Work out the finished part from the listing and answer in its coordinate system (mm). A direction names the side the tool comes from. Give positions to 0.01 mm unless a question says otherwise; leave off trailing zeros. Loops run counter-clockwise (first coordinate to the right, second up) from the corner with the lowest first, then second, coordinate; pieces in that order, holes last. Notation, with made-up numbers: M -32,53 L -22,53 A22 ccw -22,92 Z; hole C -23,23.5 d2. An arc over 180 degrees is marked long. Use a Markdown table: item, result.
```python
from build123d import *

# Parameters (mm, degrees)
SKETCH1_R           = 2.05
BOSS_EXTRUDE1_DEPTH = 170
BOSS_EXTRUDE3_START = 10
SKETCH1_3_R         = 2.05
BOSS_EXTRUDE3_DEPTH = 151
SKETCH3_R           = 2.1
SKETCH3_W           = 22.5
SKETCH3_H           = 12
CUT_EXTRUDE1_DEPTH  = 178.649984239


with BuildPart() as part:
    # Sketch1 → Boss-Extrude1 (new body)
    with BuildSketch(Plane.XY):
        Polygon((-50, 5), (50, 5), (50, -5), (50, -7.63), (-50, -7.63), (-50, -5), align=None)
        with Locations((-37.5, 0)):
            Circle(SKETCH1_R, mode=Mode.SUBTRACT)
        with Locations((-7.5, 0)):
            Circle(SKETCH1_R, mode=Mode.SUBTRACT)
        with Locations((7.5, 0)):
            Circle(SKETCH1_R, mode=Mode.SUBTRACT)
        with Locations((37.5, 0)):
            Circle(SKETCH1_R, mode=Mode.SUBTRACT)
    extrude(amount=BOSS_EXTRUDE1_DEPTH)

    # Sketch1<3> → Boss-Extrude3 (add)
    with BuildSketch(Plane.XY.offset(BOSS_EXTRUDE3_START)):
        with Locations((-37.5, 0)):
            Circle(SKETCH1_3_R)
        with Locations((-7.5, 0)):
            Circle(SKETCH1_3_R)
        with Locations((7.5, 0)):
            Circle(SKETCH1_3_R)
        with Locations((37.5, 0)):
            Circle(SKETCH1_3_R)
    extrude(amount=BOSS_EXTRUDE3_DEPTH)

    # Sketch3 → Cut-Extrude1 (cut, through all)
    with BuildSketch(Plane(origin=(0, 5, 0), x_dir=(1, 0, 0), z_dir=(0, 1, 0))):
        with Locations(Location((0, -85, 0), (0, 0, 270))):
            Circle(SKETCH3_R)
        with Locations(Location((13, -125, 0), (0, 0, 270))):
            Circle(SKETCH3_R)
        with Locations(Location((-13, -125, 0), (0, 0, 270))):
            Circle(SKETCH3_R)
        with Locations((0, -155)):
            Rectangle(SKETCH3_W, SKETCH3_H)
    extrude(amount=-CUT_EXTRUDE1_DEPTH, mode=Mode.SUBTRACT)


solid = part.part
```
(1) Given P1, Ø3.5, axis at x = -7.5, y = 0, coming from the -Z side, flat-ended and moving along its own axis, determine where the tip first touches the part or whether it passes through.
Entries:
| item | result |
|---|---|
| P1 | stops at z = 10 |
(2) A cutting plane is placed at D-D (x = 37.5). Write down the section's boundary in (y, z), and give its area (3 significant figures).
Entries:
| item | result |
|---|---|
| outline | M -7.63,0 L -2.05,0 L -2.05,10 L 2.05,10 L 2.05,0 L 5,0 L 5,170 L 2.05,170 L 2.05,161 L -2.05,161 L -2.05,170 L -7.63,170 Z |
| area | 2,070 mm² |
(3) Consider probe 1 along Y at (x, z) = (7.5, 2.5); probe 2 along Z at (x, y) = (-10, -4.25); probe 3 along X at (y, z) = (-2.25, 84). Determine where each line is inside the solid, lowest interval first. Write a range as [from, to].
Entries:
| item | result |
|---|---|
| probe 1 | y = [-7.63, -2.05], [2.05, 5] |
| probe 2 | z = [0, 149], [161, 170] |
| probe 3 | x = [-50, -1.85], [1.85, 50] |
(4) A cutting plane is placed at B-B (y = -5). Write down the section's boundary in (x, z), and give its area (3 significant figures).
Entries:
| item | result |
|---|---|
| outline | M -50,0 L 50,0 L 50,170 L -50,170 Z; hole C -13,125 d4.2; hole M -11.25,149 L 11.25,149 L 11.25,161 L -11.25,161 Z; hole C 0,85 d4.2; hole C 13,125 d4.2 |
| area | 16,700 mm² |
(5) A cutting plane is placed at A-A (x = 13). Write down the section's boundary in (y, z), and give its area (3 significant figures).
Entries:
| item | result |
|---|---|
| outline | M -7.63,0 L 5,0 L 5,122.9 L -7.63,122.9 Z; M -7.63,127.1 L 5,127.1 L 5,170 L -7.63,170 Z |
| area | 2,090 mm² |
(6) Which of the six approach directions +Z, -Z, +X, -X, +Y, -Y give full straight-line access (tool end or side, diameter ignored) to faces 4 (the flat face through (37, 0, 161)), 5 (the flat face through (50, -1, 84)), 6 (the flat face through (-12, 5, 84)), 7 (the flat face through (0, -1, 161)), 8 (the flat face through (7, 0, 10))?
Entries:
| item | result |
|---|---|
| face 4 | +Z |
| face 5 | +Z, -Z, +X, +Y, -Y |
| face 6 | +Z, -Z, +X, -X, +Y |
| face 7 | +Y, -Y |
| face 8 | -Z |
(7) A cutting plane is placed at C-C (x = -7.5). Write down the section's boundary in (y, z), and give its area (3 significant figures).
Entries:
| item | result |
|---|---|
| outline | M -7.63,0 L -2.05,0 L -2.05,10 L 2.05,10 L 2.05,0 L 5,0 L 5,149 L -7.63,149 Z; M -7.63,161 L -2.05,161 L -2.05,170 L -7.63,170 Z; M 2.05,161 L 5,161 L 5,170 L 2.05,170 Z |
| area | 1,920 mm² |
(8) The mould has two halves that part along Z. Classify faces 1 (the cylindrical face through (-9.55, 0.09, 4.93)), 2 (the cylindrical face through (13.631, -1.227, 127.003)), 3 (the flat face through (1, -1, 0)): released by +Z, released by -Z, zero draft, split by the parting line, or undercut.
Entries:
| item | result |
|---|---|
| face 1 | zero draft |
| face 2 | undercut |
| face 3 | released by -Z |
